Autodesk Inventor part; units mm, degrees
ref_plane "YZ Plane" through (0, 0, 0) normal (1, 0, 0) x (0, 1, 0)
ref_plane "XZ Plane" through (0, 0, 0) normal (0, 1, 0) x (-1, 0, 0)
ref_plane "XY Plane" through (0, 0, 0) normal (0, 0, 1) x (1, 0, 0)
sketch "Sketch1" plane through (0, 0, 0) normal (0, 1, 0) x (-1, 0, 0)
  line L0 (0, 0) -> (40, 0)
  line L1 (40, 0) -> (40, -35)
  line L2 (40, -35) -> (0, -35)
  line L3 (0, -35) -> (0, 0)
  dimension "d0" = 40
  dimension "d1" = 35
extrude "Extrusion1" add sketch "Sketch1" along normal blind 6
sketch "Sketch2" plane through (0, 6, 0) normal (0, 1, 0) x (1, 0, 0)
  line L0 (-40, 35) -> (-40, 0)
  line L1 (-40, 0) -> (-30, 0)
  line L2 (-40, 0) -> (0, 0)
  line L3 (-30, 0) -> (-20, 0)
  line L4 (-20, 0) -> (-20, -6)
  line L5 (-20, -6) -> (-30, -6)
  line L6 (-30, -6) -> (-30, 0)
  line L7 (-30, 35) -> (-20, 35)
  line L8 (-20, 35) -> (-20, 41)
  line L9 (-20, 41) -> (-30, 41)
  line L10 (-30, 41) -> (-30, 35)
  dimension "d4" = 10
  dimension "d5" = 10
  dimension "d6" = 6
  dimension "d7" = 10
  dimension "d8" = 6
extrude "Extrusion2" add sketch "Sketch2" against normal blind 6
pattern_linear "Rectangular Pattern1" count 2 spacing 20 along (1, 0, 0) of "Extrusion2"
properties part number "e_arm holder 1"
The listing builds one solid part. Answer for the finished solid, in the listing's coordinates (mm). A direction names the side the tool comes from. Round coordinates to 2 decimals unless told otherwise and drop trailing zeros. Write each loop counter-clockwise with the first axis right and the second up, starting at its lowest first coordinate (ties: lowest second). Pieces come first, ordered by that corner, then holes. Notation, with made-up numbers: M 77,-36.5 L 92,-36.5 A21 ccw 92,2.5 Z; hole C 73.25,17 d1. An arc over 180 degrees is marked long. Write each question's results on one line, items separated by ' | '. Start each with the question number.
(1) Determine the mould class of faces 6 (the flat face through (-15, 3, -35)), 7 (the flat face through (-20, 0, -17)), 8 (the flat face through (-20, 3, 3)), 9 (the flat face through (-30, 3, 3)) for opening direction X: +X half, -X half, draft (parallel to the pull), parting line (faces both ways), or undercut.
(2) The part is cut by section B-B, the plane x = -35. Write down the section's boundary in (y, z), and give its area (3 significant figures).
(3) Each of these flat-tipped pins is pushed along its axis until it touches: P1, Ø3, axis at x = -33, y = 2, coming from the -Z side; P2, Ø3, axis at x = -36, y = 3, coming from the +Z side; P3, Ø1.8, axis at y = 4, z = -38, coming from the -X side. Where does it stop, or does it pass through?
(4) For faces 1 (the flat face through (-10, 3, 3)), 2 (the flat face through (-30, 3, -38)), 3 (the flat face through (-25, 3, -41)), 4 (the flat face through (-35, 3, 0)), 5 (the flat face through (-10, 3, -38)), determine the directions among +Z, -Z, +X, -X, +Y, -Y from which every point of the face is accessible in a straight line to the end or side of a thin tool.
(5) Find the intervals of material crossed by line 1 (X direction, y = 1.6, z = 1); line 2 (Z direction, x = -35, y = 3.3), in increasing order.
(6) The part is cut by section A-A, the plane y = 4.6. Write down the section's boundary in (x, z).
Worked answers:
1) face 6: undercut | face 7: draft | face 8: undercut | face 9: -X half
2) outline: M 0,-35 L 6,-35 L 6,0 L 0,0 Z | area: 210 mm²
3) P1: stops at z = -35 | P2: stops at z = 0 | P3: stops at x = -30
4) face 1: +Z, +Y, -Y | face 2: -Z, -X, +Y, -Y | face 3: -Z, +X, -X, +Y, -Y | face 4: +Z, -X, +Y, -Y | face 5: -Z, +Y, -Y
5) line 1: x = -30 to -20, -10 to 0 | line 2: z = -35 to 0
6) outline: M -40,-35 L -30,-35 L -30,-41 L -20,-41 L -20,-35 L -10,-35 L -10,-41 L 0,-41 L 0,6 L -10,6 L -10,0 L -20,0 L -20,6 L -30,6 L -30,0 L -40,0 Z
